```python
from build123d import *

# Parameters (mm, degrees)
CROQUIS1_R              = 1.75
CROQUIS1_R_2            = 1.05
CROQUIS1_R_3            = 1.65
CROQUIS1_R_4            = 7
CROQUIS1_R_5            = 1.5
CROQUIS1_W              = 20.5
CROQUIS1_H              = 9.25
CROQUIS1_W_2            = 3.8
CROQUIS1_H_2            = 2.3
CROQUIS1_W_3            = 6
CROQUIS1_H_3            = 20
CROQUIS1_W_4            = 47.88
SALIENTE_EXTRUIR1_DEPTH = 2


with BuildPart() as part:
    # Croquis1 → Saliente-Extruir1 (new body)
    with BuildSketch(Plane(origin=(0, 0, 0), x_dir=(1, 0, 0), z_dir=(0, 1, 0))):
        with BuildLine():
            Line((-49.462248263, 45), (-49.462248263, 14))
            Line((-49.462248263, 14), (25.537751737, 14))
            Line((25.537751737, 14), (25.537751737, 45))
            Line((25.537751737, 45), (40.037751737, 45))
            Line((40.037751737, 45), (40.037751737, 14))
            Line((40.037751737, 14), (66.037751737, 14))
            Line((66.037751737, 14), (66.037751737, 45))
            Line((66.037751737, 45), (80.537751737, 45))
            ThreePointArc((80.537751737, 45), (84.073285643, 43.535533906), (85.537751737, 40))
            ThreePointArc((85.537751737, 40), (79.612228902, 28.069677764), (77.037751737, 15))
            Line((77.037751737, 15), (77.037751737, -15))
            ThreePointArc((77.037751737, -15), (79.612228902, -28.069677764), (85.537751737, -40))
            ThreePointArc((85.537751737, -40), (84.073285643, -43.535533906), (80.537751737, -45))
            Line((80.537751737, -45), (66.037751737, -45))
            Line((66.037751737, -45), (66.037751737, -14))
            Line((66.037751737, -14), (40.037751737, -14))
            Line((40.037751737, -14), (40.037751737, -45))
            Line((40.037751737, -45), (25.537751737, -45))
            Line((25.537751737, -45), (25.537751737, -14))
            Line((25.537751737, -14), (-49.462248263, -14))
            Line((-49.462248263, -14), (-49.462248263, -45))
            ThreePointArc((-49.462248263, -45), (-63.604383887, -39.142135624), (-69.462248263, -25))
            Line((-69.462248263, -25), (-69.462248263, 25))
            ThreePointArc((-69.462248263, 25), (-63.604383887, 39.142135624), (-49.462248263, 45))
        make_face()
        with Locations(Location((-58.462248263, -14, 0), (0, 0, 270))):
            Circle(CROQUIS1_R, mode=Mode.SUBTRACT)
        with Locations(Location((-58.462248263, 14, 0), (0, 0, 90))):
            Circle(CROQUIS1_R, mode=Mode.SUBTRACT)
        with Locations(Location((71.365251737, 0, 0), (0, 0, 270))):
            Circle(CROQUIS1_R_2, mode=Mode.SUBTRACT)
        with Locations(Location((47.465251737, 0, 0), (0, 0, 270))):
            Circle(CROQUIS1_R_2, mode=Mode.SUBTRACT)
        with Locations(Location((-43.462248263, 0, 0), (0, 0, 270))):
            Circle(CROQUIS1_R_3, mode=Mode.SUBTRACT)
        with Locations(Location((12.417751737, 0, 0), (0, 0, 270))):
            Circle(CROQUIS1_R_3, mode=Mode.SUBTRACT)
        with Locations(Location((-58.462248263, 0, 0), (0, 0, 270))):
            Circle(CROQUIS1_R_4, mode=Mode.SUBTRACT)
        with Locations(Location((42.037751737, 0, 0), (0, 0, 270))):
            Circle(CROQUIS1_R_5, mode=Mode.SUBTRACT)
        with Locations((59.415251737, 0)):
            Rectangle(CROQUIS1_W, CROQUIS1_H, mode=Mode.SUBTRACT)
        with Locations((30.037751737, 41.35)):
            Rectangle(CROQUIS1_W_2, CROQUIS1_H_2, mode=Mode.SUBTRACT)
        with Locations((76.137751737, 41.35)):
            Rectangle(CROQUIS1_W_2, CROQUIS1_H_2, mode=Mode.SUBTRACT)
        with Locations((76.137751737, -41.35)):
            Rectangle(CROQUIS1_W_2, CROQUIS1_H_2, mode=Mode.SUBTRACT)
        with Locations((30.037751737, -41.35)):
            Rectangle(CROQUIS1_W_2, CROQUIS1_H_2, mode=Mode.SUBTRACT)
        with Locations((33.037751737, 0)):
            Rectangle(CROQUIS1_W_3, CROQUIS1_H_3, mode=Mode.SUBTRACT)
        with Locations((-15.522248263, 0)):
            Rectangle(CROQUIS1_W_4, CROQUIS1_H_3, mode=Mode.SUBTRACT)
    extrude(amount=SALIENTE_EXTRUIR1_DEPTH)


solid = part.part
```
Build history of the part. All positions in model axes, mm. A direction names the side the tool comes from. Give positions to 0.01 mm unless a question says otherwise; leave off trailing zeros. Order: outer loops, then holes, each group sorted by start corner. A loop starts at its lowest first (then second) coordinate and runs counter-clockwise, first axis right, second up. Notation, with made-up numbers: M 76,30.5 L 129,30.5 A35 cw 129,65.5 Z; hole C -23.75,-28.75 d5. An arc over 180 degrees is marked long. Write item = value, one per line. Start each with the question number.
(1) Which spindle directions (+Z, -Z, +X, -X, +Y, -Y) get a long thin tool onto all of the face, cutting with end or side? Do faces 4 (the cylindrical face through (-44.926, 0.986, 0.761)), 5 (the cylindrical face through (79.55, 0.99, 27.89)). Say none if no direction does.
(2) Probe L1, parallel to X at y = 1.1, z = 7.5; L2, parallel to Z at x = 76.5, y = 1.1; L3, parallel to Z at x = 31, y = 0.7. List the from-to ranges inside material, lowest first. Write a range as [from, to].
(3) Pin check, flat tips, straight feed: pin 1 Ø0.6 at (x, y) = (58.5, 1.5) entering from -Z; pin 2 Ø0.6 at (y, z) = (0.5, 24.5) entering from +X. Stop position of each tip, or through.
(4) Slice it at A-A on x = 54.5. Write the cut outline in (y, z) (3 decimals), plus the area to 3 significant figures.
(5) Slice it at C-C on x = -21.5. Write the cut outline in (y, z).
(6) Slice it at D-D on x = 17.5. Write the cut outline in (y, z), plus the area to 3 significant figures.
(7) Two-plate mould, pull along Z, no slides. Class faces 1 (the cylindrical face through (-63.448, 0.986, 39.297)), 2 (the cylindrical face through (-63.759, 0.986, -38.986)), 3 (the cylindrical face through (-51.52, 0.99, -0.91)): released by +Z, released by -Z, zero draft, split by the parting line, or undercut.
(8) Slice it at B-B on z = 35.5. Write the cut outline in (x, y).
Responses:
q1.face_4 = +Y, -Y
q1.face_5 = +X, +Y, -Y
q2.L1 = [-69.46, -39.46], [8.42, 30.04], [36.04, 77.04]
q2.L2 = [-45, -42.5], [-40.2, 40.2], [42.5, 45]
q2.L3 = [-45, -42.5], [-40.2, -10], [10, 40.2], [42.5, 45]
q3.pin_1 = -14
q3.pin_2 = 78.62
q4.outline = M 0,-14 L 2,-14 L 2,-4.625 L 0,-4.625 Z; M 0,4.625 L 2,4.625 L 2,14 L 0,14 Z
q4.area = 37.5 mm2
q5.outline = M 0,-14 L 2,-14 L 2,-10 L 0,-10 Z; M 0,10 L 2,10 L 2,14 L 0,14 Z
q6.outline = M 0,-14 L 2,-14 L 2,14 L 0,14 Z
q6.area = 56.0 mm2
q7.face_1 = released by +Z
q7.face_2 = released by -Z
q7.face_3 = undercut
q8.outline = M -66.48,0 L -49.46,0 L -49.46,2 L -66.48,2 Z; M 25.54,0 L 40.04,0 L 40.04,2 L 25.54,2 Z; M 66.04,0 L 82.83,0 L 82.83,2 L 66.04,2 Z
